Source: CAD feature listing. Evaluate the final solid. Frame: model axes, mm. A direction names the side the tool comes from. Coordinates: 2 decimals unless noted, no trailing zeros. Order: outer loops, then holes, each group sorted by start corner. A loop starts at its lowest first (then second) coordinate and runs counter-clockwise, first axis right, second up.
```python
from build123d import *

# Parameters (mm, degrees)
F0_R         = 11.1
F1_DEPTH     = 6
F2_C1_SIZE2  = 3
F2_C1_SIZE   = 1.7320508076
F2_C2_SIZE2  = 3
F2_C2_SIZE   = 1.7320508076
F2_C3_SIZE2  = 3
F2_C3_SIZE   = 1.7320508076
F2_C4_SIZE2  = 3
F2_C4_SIZE   = 1.7320508076
F2_C5_SIZE2  = 1.7320508076
F2_C5_SIZE   = 3
F2_C6_SIZE2  = 3
F2_C6_SIZE   = 1.7320508076
F2_C7_SIZE2  = 1.7320508076
F2_C7_SIZE   = 3
F2_C8_SIZE2  = 3
F2_C8_SIZE   = 1.7320508076
F2_C9_SIZE2  = 1.7320508076
F2_C9_SIZE   = 3
F2_C10_SIZE2 = 3
F2_C10_SIZE  = 1.7320508076
F2_C11_SIZE2 = 3
F2_C11_SIZE  = 1.7320508076
F2_C12_SIZE2 = 3
F2_C12_SIZE  = 1.7320508076
F2_C13_SIZE2 = 1.7320508076
F2_C13_SIZE  = 3
F2_C14_SIZE2 = 3
F2_C14_SIZE  = 1.7320508076
F2_C15_SIZE2 = 3
F2_C15_SIZE  = 1.7320508076
F2_C16_SIZE2 = 3
F2_C16_SIZE  = 1.7320508076
F2_C17_SIZE2 = 1.7320508076
F2_C17_SIZE  = 3
F2_C18_SIZE2 = 3
F2_C18_SIZE  = 1.7320508076
F2_C19_SIZE2 = 3
F2_C19_SIZE  = 1.7320508076
F2_C20_SIZE2 = 3
F2_C20_SIZE  = 1.7320508076
F2_C21_SIZE2 = 1.7320508076
F2_C21_SIZE  = 3
F2_C22_SIZE2 = 3
F2_C22_SIZE  = 1.7320508076
F2_C23_SIZE2 = 3
F2_C23_SIZE  = 1.7320508076
F2_C24_SIZE2 = 3
F2_C24_SIZE  = 1.7320508076
F3_R         = 1


with BuildPart() as f1:
    # F0 (on Top) → F1 (new body)
    with BuildSketch(Plane.XY):
        with BuildLine():
            Line((8.3388454559, 22.1051900243), (0, 45))
            Line((0, 45), (-8.3388454559, 22.1051900243))
            ThreePointArc((-8.3388454559, 22.1051900243), (-7.55, 13.0769835971), (-14.9742333886, 18.2742470152))
            Line((-14.9742333886, 18.2742470152), (-38.9711431703, 22.5))
            Line((-38.9711431703, 22.5), (-23.3130788445, 3.8309430091))
            ThreePointArc((-23.3130788445, 3.8309430091), (-15.1, 0), (-23.3130788445, -3.8309430091))
            Line((-23.3130788445, -3.8309430091), (-38.9711431703, -22.5))
            Line((-38.9711431703, -22.5), (-14.9742333886, -18.2742470152))
            ThreePointArc((-14.9742333886, -18.2742470152), (-7.55, -13.0769835971), (-8.3388454559, -22.1051900243))
            Line((-8.3388454559, -22.1051900243), (0, -45))
            Line((0, -45), (8.3388454559, -22.1051900243))
            ThreePointArc((8.3388454559, -22.1051900243), (7.55, -13.0769835971), (14.9742333886, -18.2742470152))
            Line((14.9742333886, -18.2742470152), (38.9711431703, -22.5))
            Line((38.9711431703, -22.5), (23.3130788445, -3.8309430091))
            ThreePointArc((23.3130788445, -3.8309430091), (15.1, 0), (23.3130788445, 3.8309430091))
            Line((23.3130788445, 3.8309430091), (38.9711431703, 22.5))
            Line((38.9711431703, 22.5), (14.9742333886, 18.2742470152))
            ThreePointArc((14.9742333886, 18.2742470152), (7.55, 13.0769835971), (8.3388454559, 22.1051900243))
        make_face()
        Circle(F0_R, mode=Mode.SUBTRACT)
    extrude(amount=F1_DEPTH)

    # F2: chamfer of 3 x 1.7320508076 on 24 edges, made by hand

    # F2_c1
    f2_c1_edges = [f1.edges().sort_by_distance(p)[0] for p in [
        (31.1421110074, 13.1654715045, 0),
    ]]
    f2_c1_side = f1.faces().sort_by_distance((31.1421110074, 13.1654715045, 0.0346410162))[0]
    chamfer(f2_c1_edges, length=F2_C1_SIZE, length2=F2_C1_SIZE2, reference=f2_c1_side)

    # F2_c2
    f2_c2_edges = [f1.edges().sort_by_distance(p)[0] for p in [
        (31.1421110074, 13.1654715045, 6),
    ]]
    f2_c2_side = f1.faces().sort_by_distance((31.1421110074, 13.1654715045, 5.9653589838))[0]
    chamfer(f2_c2_edges, length=F2_C2_SIZE, length2=F2_C2_SIZE2, reference=f2_c2_side)

    # F2_c3
    f2_c3_edges = [f1.edges().sort_by_distance(p)[0] for p in [
        (24.6756919125, 19.9826322901, 0),
    ]]
    f2_c3_side = f1.faces().sort_by_distance((24.6816996097, 19.9485162005, 0))[0]
    chamfer(f2_c3_edges, length=F2_C3_SIZE, length2=F2_C3_SIZE2, reference=f2_c3_side)

    # F2_c4
    f2_c4_edges = [f1.edges().sort_by_distance(p)[0] for p in [
        (24.6756919125, 19.9826322901, 6),
    ]]
    f2_c4_side = f1.faces().sort_by_distance((24.6756919125, 19.9826322901, 5.9653589838))[0]
    chamfer(f2_c4_edges, length=F2_C4_SIZE, length2=F2_C4_SIZE2, reference=f2_c4_side)

    # F2_c5
    f2_c5_edges = [f1.edges().sort_by_distance(p)[0] for p in [
        (4.169422728, 33.5525950122, 0),
    ]]
    f2_c5_side = f1.faces().sort_by_distance((4.136873479, 33.5407397857, 0))[0]
    chamfer(f2_c5_edges, length=F2_C5_SIZE, length2=F2_C5_SIZE2, reference=f2_c5_side)

    # F2_c6
    f2_c6_edges = [f1.edges().sort_by_distance(p)[0] for p in [
        (4.169422728, 33.5525950122, 6),
    ]]
    f2_c6_side = f1.faces().sort_by_distance((4.169422728, 33.5525950122, 5.9653589838))[0]
    chamfer(f2_c6_edges, length=F2_C6_SIZE, length2=F2_C6_SIZE2, reference=f2_c6_side)

    # F2_c7
    f2_c7_edges = [f1.edges().sort_by_distance(p)[0] for p in [
        (-4.9676212415, 31.3610921973, 0),
    ]]
    f2_c7_side = f1.faces().sort_by_distance((-4.9350719925, 31.3492369708, 0))[0]
    chamfer(f2_c7_edges, length=F2_C7_SIZE, length2=F2_C7_SIZE2, reference=f2_c7_side)

    # F2_c8
    f2_c8_edges = [f1.edges().sort_by_distance(p)[0] for p in [
        (-4.9676212415, 31.3610921973, 6),
    ]]
    f2_c8_side = f1.faces().sort_by_distance((-4.9676212415, 31.3610921973, 5.9653589838))[0]
    chamfer(f2_c8_edges, length=F2_C8_SIZE, length2=F2_C8_SIZE2, reference=f2_c8_side)

    # F2_c9
    f2_c9_edges = [f1.edges().sort_by_distance(p)[0] for p in [
        (-26.9726882794, 20.3871235076, 0),
    ]]
    f2_c9_side = f1.faces().sort_by_distance((-26.9786959766, 20.353007418, 0))[0]
    chamfer(f2_c9_edges, length=F2_C9_SIZE, length2=F2_C9_SIZE2, reference=f2_c9_side)

    # F2_c10
    f2_c10_edges = [f1.edges().sort_by_distance(p)[0] for p in [
        (-26.9726882794, 20.3871235076, 6),
    ]]
    f2_c10_side = f1.faces().sort_by_distance((-26.9726882794, 20.3871235076, 5.9653589838))[0]
    chamfer(f2_c10_edges, length=F2_C10_SIZE, length2=F2_C10_SIZE2, reference=f2_c10_side)

    # F2_c11
    f2_c11_edges = [f1.edges().sort_by_distance(p)[0] for p in [
        (-29.643313154, 11.3784599071, 0),
    ]]
    f2_c11_side = f1.faces().sort_by_distance((-29.6167716023, 11.4007207704, 0))[0]
    chamfer(f2_c11_edges, length=F2_C11_SIZE, length2=F2_C11_SIZE2, reference=f2_c11_side)

    # F2_c12
    f2_c12_edges = [f1.edges().sort_by_distance(p)[0] for p in [
        (-29.643313154, 11.3784599071, 6),
    ]]
    f2_c12_side = f1.faces().sort_by_distance((-29.643313154, 11.3784599071, 5.9653589838))[0]
    chamfer(f2_c12_edges, length=F2_C12_SIZE, length2=F2_C12_SIZE2, reference=f2_c12_side)

    # F2_c13
    f2_c13_edges = [f1.edges().sort_by_distance(p)[0] for p in [
        (-31.1421110074, -13.1654715045, 0),
    ]]
    f2_c13_side = f1.faces().sort_by_distance((-31.1155694557, -13.1877323678, 0))[0]
    chamfer(f2_c13_edges, length=F2_C13_SIZE, length2=F2_C13_SIZE2, reference=f2_c13_side)

    # F2_c14
    f2_c14_edges = [f1.edges().sort_by_distance(p)[0] for p in [
        (-31.1421110074, -13.1654715045, 6),
    ]]
    f2_c14_side = f1.faces().sort_by_distance((-31.1421110074, -13.1654715045, 5.9653589838))[0]
    chamfer(f2_c14_edges, length=F2_C14_SIZE, length2=F2_C14_SIZE2, reference=f2_c14_side)

    # F2_c15
    f2_c15_edges = [f1.edges().sort_by_distance(p)[0] for p in [
        (-24.6756919125, -19.9826322901, 0),
    ]]
    f2_c15_side = f1.faces().sort_by_distance((-24.6816996097, -19.9485162005, 0))[0]
    chamfer(f2_c15_edges, length=F2_C15_SIZE, length2=F2_C15_SIZE2, reference=f2_c15_side)

    # F2_c16
    f2_c16_edges = [f1.edges().sort_by_distance(p)[0] for p in [
        (-24.6756919125, -19.9826322901, 6),
    ]]
    f2_c16_side = f1.faces().sort_by_distance((-24.6756919125, -19.9826322901, 5.9653589838))[0]
    chamfer(f2_c16_edges, length=F2_C16_SIZE, length2=F2_C16_SIZE2, reference=f2_c16_side)

    # F2_c17
    f2_c17_edges = [f1.edges().sort_by_distance(p)[0] for p in [
        (-4.169422728, -33.5525950122, 0),
    ]]
    f2_c17_side = f1.faces().sort_by_distance((-4.136873479, -33.5407397857, 0))[0]
    chamfer(f2_c17_edges, length=F2_C17_SIZE, length2=F2_C17_SIZE2, reference=f2_c17_side)

    # F2_c18
    f2_c18_edges = [f1.edges().sort_by_distance(p)[0] for p in [
        (-4.169422728, -33.5525950122, 6),
    ]]
    f2_c18_side = f1.faces().sort_by_distance((-4.169422728, -33.5525950122, 5.9653589838))[0]
    chamfer(f2_c18_edges, length=F2_C18_SIZE, length2=F2_C18_SIZE2, reference=f2_c18_side)

    # F2_c19
    f2_c19_edges = [f1.edges().sort_by_distance(p)[0] for p in [
        (4.9676212415, -31.3610921973, 0),
    ]]
    f2_c19_side = f1.faces().sort_by_distance((4.9350719925, -31.3492369708, 0))[0]
    chamfer(f2_c19_edges, length=F2_C19_SIZE, length2=F2_C19_SIZE2, reference=f2_c19_side)

    # F2_c20
    f2_c20_edges = [f1.edges().sort_by_distance(p)[0] for p in [
        (4.9676212415, -31.3610921973, 6),
    ]]
    f2_c20_side = f1.faces().sort_by_distance((4.9676212415, -31.3610921973, 5.9653589838))[0]
    chamfer(f2_c20_edges, length=F2_C20_SIZE, length2=F2_C20_SIZE2, reference=f2_c20_side)

    # F2_c21
    f2_c21_edges = [f1.edges().sort_by_distance(p)[0] for p in [
        (26.9726882794, -20.3871235076, 0),
    ]]
    f2_c21_side = f1.faces().sort_by_distance((26.9786959766, -20.353007418, 0))[0]
    chamfer(f2_c21_edges, length=F2_C21_SIZE, length2=F2_C21_SIZE2, reference=f2_c21_side)

    # F2_c22
    f2_c22_edges = [f1.edges().sort_by_distance(p)[0] for p in [
        (26.9726882794, -20.3871235076, 6),
    ]]
    f2_c22_side = f1.faces().sort_by_distance((26.9726882794, -20.3871235076, 5.9653589838))[0]
    chamfer(f2_c22_edges, length=F2_C22_SIZE, length2=F2_C22_SIZE2, reference=f2_c22_side)

    # F2_c23
    f2_c23_edges = [f1.edges().sort_by_distance(p)[0] for p in [
        (29.643313154, -11.3784599071, 0),
    ]]
    f2_c23_side = f1.faces().sort_by_distance((29.6167716023, -11.4007207704, 0))[0]
    chamfer(f2_c23_edges, length=F2_C23_SIZE, length2=F2_C23_SIZE2, reference=f2_c23_side)

    # F2_c24
    f2_c24_edges = [f1.edges().sort_by_distance(p)[0] for p in [
        (29.643313154, -11.3784599071, 6),
    ]]
    f2_c24_side = f1.faces().sort_by_distance((29.643313154, -11.3784599071, 5.9653589838))[0]
    chamfer(f2_c24_edges, length=F2_C24_SIZE, length2=F2_C24_SIZE2, reference=f2_c24_side)

    # F3
    f3_edges = [f1.edges().sort_by_distance(p)[0] for p in [
        (-11.1, 0, 0),
        (-11.1, 0, 6),
    ]]
    fillet(f3_edges, radius=F3_R)


solid = f1.part
```
1. Section query A-A, the plane y = 0. Output: boundary loops of the cut face in (x, z).
2. Contact query for a flat-ended pin moving along its axis: P1, Ø18, axis at x = 0, y = 0, coming from the +Z side. Output: stop coordinate, or through.
3. Section query B-B, the plane x = -26. Output: boundary loops of the cut face in (y, z), plus the area to 3 significant figures.
4. Section query C-C, the plane y = 32. Output: boundary loops of the cut face in (x, z).
5. Section query D-D, the plane x = -7. Count the separate pieces of the cut face and the enclosed holes in it, plus the area to 3 significant figures.
6. Access query for faces 5 (the flat face through (26.805, -20.358, 2.982)), 6 (the flat face through (-26.01, 18.72, 0.88)), 7 (the flat face through (31.252, -13.296, 3.625)), 8 (the flat face through (26.01, -18.72, 0.88)), 9 (the flat face through (-31.252, 13.296, 3.625)). Directions: +Z, -Z, +X, -X, +Y, -Y. A direction counts if a zero-diameter tool reaches every point of the face in a straight line with its end or side. Return the directions, or none.
7. Draft query along X for faces 1 (the flat face through (-12, 3, 6)), 2 (the cylindrical face through (7.41, -13.16, 2.96)), 3 (the flat face through (23.793, -18.283, 5.146)), 4 (the flat face through (29.181, 13.194, 0.854)). Return one class per face: +X half, -X half, draft (parallel to the pull), parting line (faces both ways), or undercut.
8. Material intervals for line 1 along Y through (x, z) = (10.05, 4.25); line 2 along Y through (x, z) = (-25, 2); line 3 along X through (y, z) = (-8, 2), sorted ascending.
Answer key:
1. outline: (-15.1, 0) - (-12.1, 0) arc R1 ccw to (-11.1, 1) - (-11.1, 5) arc R1 ccw to (-12.1, 6) - (-15.1, 6) - close; (11.1, 1) arc R1 ccw to (12.1, 0) - (15.1, 0) - (15.1, 6) - (12.1, 6) arc R1 ccw to (11.1, 5) - close
2. P1: passes through
3. outline: (-20.22, 3) - (-18.46, 0) - (-11.7, 0) - (-7.03, 1.73) - (-7.03, 4.27) - (-11.7, 6) - (-17.17, 6) - (-20.22, 4.27) - close; (7.03, 3) - (9.73, 0) - (17.17, 0) - (20.22, 1.73) - (20.22, 4.27) - (17.17, 6) - (11.7, 6) - (7.03, 4.27) - close
3. area: 131 mm2
4. outline: (-4.73, 1.73) - (-1.54, 0) - (1.54, 0) - (4.73, 1.73) - (4.73, 4.27) - (1.54, 6) - (-1.54, 6) - (-4.73, 4.27) - close
5. separate pieces: 4
5. enclosed holes: 0
5. area: 86.9 mm2
6. face 5: +Z, -Z, -Y
6. face 6: -Z, +Y
6. face 7: +Z, -Z, +X
6. face 8: -Z, -Y
6. face 9: +Z, -Z, -X
7. face 1: draft
7. face 2: undercut
7. face 3: undercut
7. face 4: +X half
8. line 1: y = -12.41 to -4.71, 4.71 to 12.41
8. line 2: y = -19.45 to -5.84, 6.74 to 20.04
8. line 3: x = -26.81 to -7.69, 7.69 to 26.06
